Verification items for the finished model (mm, model axes). A direction names the side the tool comes from. Give positions to 0.01 mm unless a question says otherwise; leave off trailing zeros. Loops run counter-clockwise (first coordinate to the right, second up) from the corner with the lowest first, then second, coordinate; pieces in that order, holes last. Notation, with made-up numbers: (46, 80) - (82, 80) arc R13 cw to (82, 93) - close; hole circle Ø11 at (6.25, 55). An arc over 180 degrees is marked (long way). Use one line per item in the form item = value.
Autodesk Inventor part; units mm, degrees
ref_plane "YZ Plane" through (0, 0, 0) normal (1, 0, 0) x (0, 1, 0)
ref_plane "XZ Plane" through (0, 0, 0) normal (0, 1, 0) x (-1, 0, 0)
ref_plane "XY Plane" through (0, 0, 0) normal (0, 0, 1) x (1, 0, 0)
sketch "Sketch1" plane through (0, 0, 0) normal (0, 1, 0) x (-1, 0, 0)
  circle A0 centre (0, 0) radius 14
  dimension "d0" = 28
extrude "Extrusion1" add sketch "Sketch1" along normal blind 1
sketch "Sketch2" plane through (0, 1, 0) normal (0, 1, 0) x (1, 0, 0)
  circle A0 centre (0, 0) radius 13.25
  dimension "d3" = 26.5
extrude "Extrusion2" add sketch "Sketch2" along normal blind 3
sketch "Sketch3" plane through (0, 4, 0) normal (0, 1, 0) x (1, 0, 0)
  circle A0 centre (0, 0) radius 14
  dimension "d6" = 28
extrude "Extrusion3" add sketch "Sketch3" along normal blind 1
sketch "Sketch4" plane through (0, 5, 0) normal (0, 1, 0) x (1, 0, 0)
  circle A0 centre (-6, 0) radius 2.2
  circle A1 centre (6, 0) radius 2.2
  circle A2 centre (0, -6) radius 2.2
  circle A3 centre (0, 6) radius 2.2
  point P0 (0, 0)
  dimension "d9" = 4.4
  dimension "d10" = 6
  dimension "d11" = 4.4
  dimension "d12" = 12
  dimension "d13" = 4.4
  dimension "d14" = 6
  dimension "d15" = 4.4
  dimension "d16" = 6
hole "Hole1" at (0, 5, 6) at (-6, 5, 0) at (6, 5, 0) at (0, 5, -6) direction (0, -1, 0) diameter 4.4 end through all
properties part number "XLRotorWheel" material "ABS Plastic"
1. Scan lines: probe 1 along Z at (x, y) = (0, 1.9); probe 2 along Y at (x, z) = (7.5, 11.5). Record each from-to range of solid material in increasing order.
Result set:
probe_1 = -13.25 to -8.2, -3.8 to 3.8, 8.2 to 13.25
probe_2 = 0 to 1, 4 to 5
2. Draft check along Z on faces 3 (the cylindrical face through (-0.66, 2.46, -3.9)), 4 (the cylindrical face through (0.843, 2.465, 8.032)), 5 (the flat face through (0, 0, 0)), 6 (the cylindrical face through (12.932, 4.493, -5.362)). Enter one of: released by +Z, released by -Z, zero draft, split by the parting line, or undercut.
Result set:
face_3 = undercut
face_4 = undercut
face_5 = zero draft
face_6 = split by the parting line
3. Section check C-C, the plane x = 0. Record the cut outline in (y, z).
Result set:
outline = (0, -14) - (1, -14) - (1, -13.25) - (4, -13.25) - (4, -14) - (5, -14) - (5, -8.2) - (0, -8.2) - close; (0, -3.8) - (5, -3.8) - (5, 3.8) - (0, 3.8) - close; (0, 8.2) - (5, 8.2) - (5, 14) - (4, 14) - (4, 13.25) - (1, 13.25) - (1, 14) - (0, 14) - close
4. Section check A-A, the plane z = 0. Record the cut outline in (x, y), then the cut area to 3 significant figures.
Result set:
outline = (-14, 0) - (-8.2, 0) - (-8.2, 5) - (-14, 5) - (-14, 4) - (-13.25, 4) - (-13.25, 1) - (-14, 1) - close; (-3.8, 0) - (3.8, 0) - (3.8, 5) - (-3.8, 5) - close; (8.2, 0) - (14, 0) - (14, 1) - (13.25, 1) - (13.25, 4) - (14, 4) - (14, 5) - (8.2, 5) - close
area = 91.5 mm²
5. Depth check by flat-ended pin: pin 1 Ø1.5 at (y, z) = (3, 8) entering from +X; pin 2 Ø2.5 at (x, z) = (6, 0) entering from -Y; pin 3 Ø2 at (y, z) = (2.5, -6.5) entering from +X. Enter the tip coordinate at first touch or a pass-through.
Result set:
pin_1 = 11.09
pin_2 = through
pin_3 = 12.05
6. Section check D-D, the plane x = 5. Record the cut outline in (y, z).
Result set:
outline = (0, -13.08) - (1, -13.08) - (1, -12.27) - (4, -12.27) - (4, -13.08) - (5, -13.08) - (5, -1.96) - (0, -1.96) - close; (0, 1.96) - (5, 1.96) - (5, 13.08) - (4, 13.08) - (4, 12.27) - (1, 12.27) - (1, 13.08) - (0, 13.08) - close
7. Section check B-B, the plane y = 3. Record the cut outline in (x, z), then the cut area to 3 significant figures.
Result set:
outline = circle Ø26.5 at (0, 0); hole circle Ø4.4 at (-6, 0); hole circle Ø4.4 at (0, -6); hole circle Ø4.4 at (0, 6); hole circle Ø4.4 at (6, 0)
area = 491 mm²
8. Tool access check on faces 1 (the flat face through (0, 5, 0)), 2 (the flat face through (12.4, 4, 5.1)). Record the directions out of +Z, -Z, +X, -X, +Y, -Y that give a thin tool (end or side, any length) a straight path to the whole face; none if there is none.
Result set:
face_1 = +Z, -Z, +X, -X, +Y
face_2 = none
